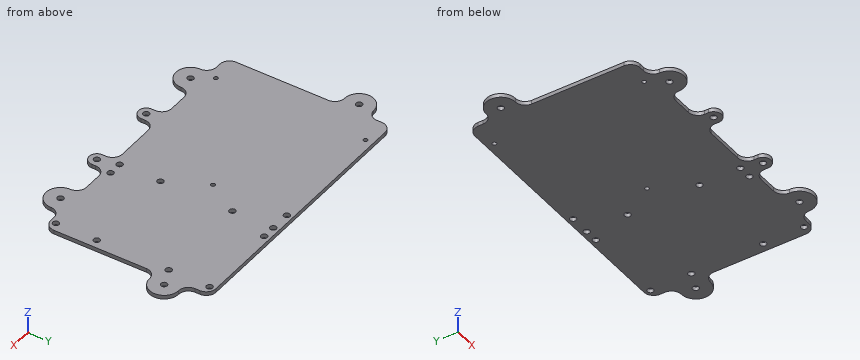
Autodesk Inventor part; units mm, degrees
ref_plane "YZ Plane" through (0, 0, 0) normal (1, 0, 0) x (0, 1, 0)
ref_plane "XZ Plane" through (0, 0, 0) normal (0, 1, 0) x (-1, 0, 0)
ref_plane "XY Plane" through (0, 0, 0) normal (0, 0, 1) x (1, 0, 0)
sketch "Skizze1" plane through (0, 0, 0) normal (0, 0, 1) x (1, 0, 0)
  line L0 (-70, 22.5) -> (-75, 22.5)
  line L1 (-75, 7.5) -> (-70, 7.5)
  line L2 (70, 22.5) -> (75, 22.5)
  line L3 (75, 7.5) -> (70, 7.5)
  arc A0 (-75, 22.5) -> (-75, 7.5) centre (-75, 15) ccw
  arc A1 (-57.5, -55) -> (-42.5, -55) centre (-50, -55) ccw
  arc A2 (75, 7.5) -> (75, 22.5) centre (75, 15) ccw
  arc A3 (42.5, -55) -> (57.5, -55) centre (50, -55) ccw
  line L4 (-70, 22.5) -> (-70, 35)
  line L5 (-70, -50) -> (-70, 7.5)
  line L6 (70, 35) -> (70, 22.5)
  line L7 (70, 7.5) -> (70, -50)
  line L8 (0, 54.5) -> (0, -82)
  line L9 (-115.5, 0) -> (115.5, 0)
  line L10 (-70, 35) -> (70, 35)
  line L11 (23, -50) -> (23, -57)
  line L12 (15, -50) -> (15, -57)
  line L13 (-15, -50) -> (-15, -57)
  line L14 (-23, -50) -> (-23, -57)
  arc A4 (15, -57) -> (23, -57) centre (19, -57) ccw
  arc A5 (-23, -57) -> (-15, -57) centre (-19, -57) ccw
  line L15 (15, -50) -> (-15, -50)
  line L16 (57.5, -50) -> (57.5, -55)
  line L17 (42.5, -55) -> (42.5, -50)
  line L18 (-42.5, -55) -> (-42.5, -50)
  line L19 (-57.5, -55) -> (-57.5, -50)
  line L20 (70, -50) -> (57.5, -50)
  line L21 (42.5, -50) -> (23, -50)
  line L22 (-23, -50) -> (-42.5, -50)
  line L23 (-57.5, -50) -> (-70, -50)
  point P0 (0, 0)
  dimension "d0" = 85
  dimension "d2" = 15
  dimension "d6" = 75
  dimension "d21" = 15
  dimension "d71" = 35
  dimension "d72" = 70
  dimension "d73" = 7
  dimension "d74" = 38
  dimension "d75" = 8
  dimension "d90" = 15
  dimension "d91" = 55
  dimension "d92" = 50
extrude "Extrusion1" add sketch "Skizze1" along normal blind 2
sketch "Skizze2" plane through (0, 0, 2) normal (0, 0, 1) x (1, 0, 0)
  arc A0 (-75, 22.5) -> (-75, 7.5) centre (-75, 15) ccw
  arc A1 (-57.5, -55) -> (-42.5, -55) centre (-50, -55) ccw
  arc A2 (75, 7.5) -> (75, 22.5) centre (75, 15) ccw
  arc A3 (42.5, -55) -> (57.5, -55) centre (50, -55) ccw
  point P0 (0, 0)
hole "Montage" at (-75, 15, 2) at (75, 15, 2) at (50, -55, 2) at (-50, -55, 2) direction (0, 0, -1) diameter 3.2 end through all
fillet "Rundung1" radius 5 16 edges at (-70, 7.5, 1) (-70, 35, 1) (-70, -50, 1) (-70, 22.5, 1) (70, 35, 1) (70, 22.5, 1) (70, 7.5, 1) (70, -50, 1) (23, -50, 1) (15, -50, 1) (-15, -50, 1) (-23, -50, 1) (57.5, -50, 1) (42.5, -50, 1) (-57.5, -50, 1) (-42.5, -50, 1)
sketch "Skizze3" plane through (0, 0, 2) normal (0, 0, 1) x (1, 0, 0)
  line L0 (0, 54.5) -> (0, -82)
  line L1 (-115.5, 0) -> (115.5, 0)
  line L2 (65.5, -26) -> (16.5, -26) construction
  line L3 (16.5, -26) -> (16.5, 32) construction
  line L4 (16.5, 32) -> (65.5, 32) construction
  line L5 (65.5, 32) -> (65.5, -26) construction
  line L6 (16.5, -47) -> (65.5, -47) construction
  line L7 (65.5, -47) -> (65.5, 11) construction
  line L8 (65.5, 11) -> (16.5, 11) construction
  line L9 (16.5, 11) -> (16.5, -47) construction
  point P0 (0, 0)
  dimension "d23" = 49
  dimension "d24" = 58
  dimension "d25" = 32
  dimension "d26" = 16.5
  dimension "d94" = 49
  dimension "d95" = 58
  dimension "d97" = 47
hole "RPi" at (65.5, -26, 2) at (16.5, -26, 2) at (65.5, 32, 2) at (16.5, 32, 2) at (16.5, 11, 2) at (65.5, 11, 2) at (65.5, -47, 2) at (16.5, -47, 2) direction (0, 0, -1) diameter 3.2 end through all
sketch "Skizze4" plane through (0, 0, 2) normal (0, 0, 1) x (1, 0, 0)
  circle A0 centre (65.5, 32) radius 1.6
  line L0 (65.5, 32) -> (23.5, 32) construction
  line L1 (23.5, 32) -> (23.5, -47) construction
  line L2 (23.5, -47) -> (65.5, -47) construction
  line L3 (65.5, -47) -> (65.5, 32) construction
  point P0 (0, 0)
  dimension "d34" = 42
  dimension "d35" = 79
hole "Jetson" at (65.5, -47, 2) at (23.5, -47, 2) at (23.5, 32, 2) direction (0, 0, -1) diameter 3.2 end through all
sketch "Skizze6" plane through (0, 0, 2) normal (0, 0, 1) x (1, 0, 0)
  line L0 (0, 54.5) -> (0, -82)
  line L1 (-115.5, 0) -> (115.5, 0)
  line L2 (62.5, -50) -> (65, -50) construction
  line L3 (65, 35) -> (-65, 35) construction
  arc A0 (15, -57) -> (23, -57) centre (19, -57) ccw
  arc A1 (-23, -57) -> (-15, -57) centre (-19, -57) ccw
  point P0 (0, 0)
  point P1 (6, 32)
  point P2 (-65, -50)
  point P3 (23, -50)
  point P4 (28, -50)
  point P5 (57.5, -50)
  dimension "d61" = 3
  dimension "d63" = 6
hole "Kameras oben" at (19, -57, 2) at (6, 32, 2) at (-19, -57, 2) direction (0, 0, -1) diameter 3.2 end through all
sketch "Skizze7" plane through (0, 0, 2) normal (0, 0, 1) x (1, 0, 0)
  line L0 (0, 54.5) -> (0, -82)
  line L1 (-115.5, 0) -> (115.5, 0)
  point P0 (0, 0)
  point P1 (-56, 31)
  point P2 (-56, -46)
  point P3 (6, -6)
  dimension "d76" = 56
  dimension "d78" = 56
  dimension "d79" = 46
  dimension "d81" = 31
  dimension "d89" = 6
  dimension "d93" = 6
hole "Mainboard" at (-56, 31, 2) at (-56, -46, 2) at (6, -6, 2) direction (0, 0, -1) diameter 2.1 end through all
properties part number "Oberplatte" material "Aluminium 6061"
Geometry check sheet. Reference: the model listing, model coordinates, mm. Give positions to 0.01 mm unless a question says otherwise; leave off trailing zeros. Loops run counter-clockwise (first coordinate to the right, second up) from the corner with the lowest first, then second, coordinate; pieces in that order, holes last. Notation, with made-up numbers: M 34,58.5 L 67,58.5 A17 cw 67,69.5 Z; hole C 28,-11.75 d4. An arc over 180 degrees is marked long. Write item = value, one per line. Start each with the question number.
1. Section check B-B, the plane z = 1.35. Give the number of separate pieces and of enclosed holes in the cut face, plus the area to 3 significant figures.
2. Section check A-A, the plane y = 15. Enter the section's corners in (x, z).
3. Section check D-D, the plane x = -26. Enter the section's corners in (y, z).
4. Go/stop test with a flat-tipped pin: P1, Ø1, axis at y = 28.5, z = 0.5, coming from the +X side. Record where the tip stops, or that it passes through.
5. Thickness scan on probe 1 along X at (y, z) = (-26, 1.45); probe 2 along Y at (x, z) = (50, 1.35); probe 3 along Y at (x, z) = (-75, 1.25). Record the ranges inside material, lowest first.
6. Section check C-C, the plane y = 0. Enter the section's corners in (x, z).
Values follow:
q1.separate_pieces = 1
q1.enclosed_holes = 20
q1.area = 12,600 mm^2
q2.outline = M -82.5,0 L -76.6,0 L -76.6,2 L -82.5,2 Z; M -73.4,0 L 73.4,0 L 73.4,2 L -73.4,2 Z; M 76.6,0 L 82.5,0 L 82.5,2 L 76.6,2 Z
q3.outline = M -50.42,0 L 35,0 L 35,2 L -50.42,2 Z
q4.P1 = 70
q5.probe_1 = -70 to 14.9, 18.1 to 63.9, 67.1 to 70
q5.probe_2 = -62.5 to -56.6, -53.4 to 35
q5.probe_3 = 7.5 to 13.4, 16.6 to 22.5
q6.outline = M -70,0 L 70,0 L 70,2 L -70,2 Z
